from build123d import *

# Parameters (mm, degrees)
SKETCH1_R           = 0.75
SKETCH1_R_2         = 0.5
BOSS_EXTRUDE1_DEPTH = 4
SKETCH2_W           = 16.2
SKETCH2_H           = 11.98
CUT_EXTRUDE1_DEPTH  = 2


with BuildPart() as part:
    # Sketch1 → Boss-Extrude1 (new body)
    with BuildSketch(Plane.XY):
        with BuildLine():
            Line((3.1, 16.98), (-3.1, 16.98))
            ThreePointArc((-3.1, 16.98), (-6.635533906, 15.515533906), (-8.1, 11.98))
            Line((-8.1, 11.98), (-8.1, 6))
            Line((-8.1, 6), (-4.1, 6))
            Line((-4.1, 6), (-4.1, 4))
            Line((-4.1, 4), (-8.1, 4))
            Line((-8.1, 4), (-8.1, 2))
            ThreePointArc((-8.1, 2), (-7.514213562, 0.585786438), (-6.1, 0))
            Line((-6.1, 0), (6.1, 0))
            ThreePointArc((6.1, 0), (7.514213562, 0.585786438), (8.1, 2))
            Line((8.1, 2), (8.1, 4))
            Line((8.1, 4), (4.1, 4))
            Line((4.1, 4), (4.1, 6))
            Line((4.1, 6), (8.1, 6))
            Line((8.1, 6), (8.1, 11.98))
            ThreePointArc((8.1, 11.98), (6.635533906, 15.515533906), (3.1, 16.98))
        make_face()
        with Locations(Location((-5.35, 2, 0), (0, 0, 180))):
            Circle(SKETCH1_R, mode=Mode.SUBTRACT)
        with Locations(Location((-5.1, 13.98, 0), (0, 0, 180))):
            Circle(SKETCH1_R_2, mode=Mode.SUBTRACT)
        with Locations(Location((-5.35, 8.5, 0), (0, 0, 180))):
            Circle(SKETCH1_R, mode=Mode.SUBTRACT)
        with Locations((5.35, 8.5)):
            Circle(SKETCH1_R, mode=Mode.SUBTRACT)
        with Locations((5.1, 13.98)):
            Circle(SKETCH1_R_2, mode=Mode.SUBTRACT)
        with Locations((5.35, 2)):
            Circle(SKETCH1_R, mode=Mode.SUBTRACT)
    extrude(amount=BOSS_EXTRUDE1_DEPTH)

    # Sketch2 → Cut-Extrude1 (cut)
    with BuildSketch(Plane.XY):
        with Locations((0, 5.99)):
            Rectangle(SKETCH2_W, SKETCH2_H)
    extrude(amount=CUT_EXTRUDE1_DEPTH, mode=Mode.SUBTRACT)


solid = part.part
Work out the finished part from the listing and answer in its coordinate system (mm). A direction names the side the tool comes from. Round coordinates to 2 decimals unless told otherwise and drop trailing zeros. Write each loop counter-clockwise with the first axis right and the second up, starting at its lowest first coordinate (ties: lowest second). Pieces come first, ordered by that corner, then holes. Notation, with made-up numbers: (-3.5, 5.5) -> (29.5, 5.5) arc R33 cw to (29.5, 37.5) -> close; hole circle Ø9 at (0.25, 49). An arc over 180 degrees is marked (long way). Answer as CSV lines item,"result". Start each with the question number.
(1) The mould has two halves that part along Y. Classify faces 4 (the flat face through (-6, 4, 3)), 5 (the cylindrical face through (6.67, 15.48, 1.97)), 6 (the flat face through (8.1, 9, 3)): +Y half, -Y half, draft (parallel to the pull), parting line (faces both ways), or undercut.
(2) Find the intervals of material crossed by probe 1 along Y at (x, z) = (5.1, 3.15); probe 2 along Y at (x, z) = (-5.35, 3.45); probe 3 along X at (y, z) = (13.75, 1.8), in increasing order.
(3) Each of these flat-tipped pins is pushed along its axis until it touches: pin 1 (0.6 mm diameter, centred on y = 5, z = 3, fed in from +X); pin 2 (0.6 mm diameter, centred on x = 6.5, z = 3, fed in from +Y); pin 3 (1.6 mm diameter, centred on x = -2.5, z = 1, fed in from -Y). Where does it stop, or does it pass through?
(4) The part is cut by section D-D, the plane x = 7. Give the vertices of the cut face in (y, z).
(5) The part is cut by section C-C, the plane z = 2.85. Give the vertices of the cut face in (x, y).
(6) The part is cut by section A-A, the plane y = 13.98. Give the vertices of the cut face in (x, z), then the cut area to 3 significant figures.
(7) A tool of negligible diameter and unlimited length cuts with its end or side. For faces 1 (the cylindrical face through (5.8, 2.6, 3)), 2 (the flat face through (-4.1, 5, 3)), 3 (the flat face through (4.1, 5, 3)), from which of +Z, -Z, +X, -X, +Y, -Y can it reach the whole face along a straight path? Write none if from no direction.
(8) The part is cut by section B-B, the plane x = -5.35. Give the vertices of the cut face in (y, z), then the cut area to 3 significant figures.
Output values:
1,face 4,"undercut"
1,face 5,"+Y half"
1,face 6,"draft"
2,probe 1,"y = 0 to 1.29, 2.71 to 4, 6 to 7.79, 9.21 to 13.48, 14.48 to 16.56"
2,probe 2,"y = 0 to 1.25, 2.75 to 4, 6 to 7.75, 9.25 to 13.55, 14.41 to 16.45"
2,probe 3,"x = -7.78 to -5.54, -4.66 to 4.66, 5.54 to 7.78"
3,pin 1,"stops at x = 4.1"
3,pin 2,"stops at y = 15.9"
3,pin 3,"stops at y = 11.98"
4,outline,"(0.21, 2) -> (4, 2) -> (4, 4) -> (0.21, 4) -> close; (6, 2) -> (11.98, 2) -> (11.98, 0) -> (15.11, 0) -> (15.11, 4) -> (6, 4) -> close"
5,outline,"(-8.1, 2) arc R2 ccw to (-6.1, 0) -> (6.1, 0) arc R2 ccw to (8.1, 2) -> (8.1, 4) -> (4.1, 4) -> (4.1, 6) -> (8.1, 6) -> (8.1, 11.98) arc R5 ccw to (3.1, 16.98) -> (-3.1, 16.98) arc R5 ccw to (-8.1, 11.98) -> (-8.1, 6) -> (-4.1, 6) -> (-4.1, 4) -> (-8.1, 4) -> close; hole circle Ø1.5 at (-5.35, 2); hole circle Ø1.5 at (-5.35, 8.5); hole circle Ø1 at (-5.1, 13.98); hole circle Ø1.5 at (5.35, 2); hole circle Ø1.5 at (5.35, 8.5); hole circle Ø1 at (5.1, 13.98)"
6,outline,"(-7.68, 0) -> (-5.6, 0) -> (-5.6, 4) -> (-7.68, 4) -> close; (-4.6, 0) -> (4.6, 0) -> (4.6, 4) -> (-4.6, 4) -> close; (5.6, 0) -> (7.68, 0) -> (7.68, 4) -> (5.6, 4) -> close"
6,area,"53.5 mm²"
7,face 1,"+Z, -Z"
7,face 2,"+Z, -Z, -X"
7,face 3,"+Z, -Z, +X"
8,outline,"(0, 2) -> (1.25, 2) -> (1.25, 4) -> (0, 4) -> close; (2.75, 2) -> (4, 2) -> (4, 4) -> (2.75, 4) -> close; (6, 2) -> (7.75, 2) -> (7.75, 4) -> (6, 4) -> close; (9.25, 2) -> (11.98, 2) -> (11.98, 0) -> (13.55, 0) -> (13.55, 4) -> (9.25, 4) -> close; (14.41, 0) -> (16.45, 0) -> (16.45, 4) -> (14.41, 4) -> close"
8,area,"28.4 mm²"
